from build123d import *

# Parameters (mm, degrees)
F_0_5IN_SOCKET_R    = 27.94
F_0_5IN_SOCKET_R_2  = 2.1
BOSS_EXTRUDE1_DEPTH = 6.35


with BuildPart() as part:
    # 0.5in Socket → Boss-Extrude1 (new body)
    with BuildSketch(Plane(origin=(0, 0, 0), x_dir=(1, 0, 0), z_dir=(0, 1, 0))):
        with Locations(Location((0, 0, 0), (0, 0, 270))):
            Circle(F_0_5IN_SOCKET_R)
        with Locations(Location((-14.997027722, -14.997027722, 0), (0, 0, 270))):
            Circle(F_0_5IN_SOCKET_R_2, mode=Mode.SUBTRACT)
        with Locations(Location((-14.997027722, 14.997027722, 0), (0, 0, 270))):
            Circle(F_0_5IN_SOCKET_R_2, mode=Mode.SUBTRACT)
        with Locations(Location((14.997027722, 14.997027722, 0), (0, 0, 270))):
            Circle(F_0_5IN_SOCKET_R_2, mode=Mode.SUBTRACT)
        with Locations(Location((14.997027722, -14.997027722, 0), (0, 0, 270))):
            Circle(F_0_5IN_SOCKET_R_2, mode=Mode.SUBTRACT)
        with BuildLine():
            ThreePointArc((2.530034488, -14.126221239), (0, -16.891), (-2.530034488, -14.126221239))
            ThreePointArc((-2.530034488, -14.126221239), (-14.351, 0), (-2.530034488, 14.126221239))
            ThreePointArc((-2.530034488, 14.126221239), (0, 16.891), (2.530034488, 14.126221239))
            ThreePointArc((2.530034488, 14.126221239), (14.351, 0), (2.530034488, -14.126221239))
        make_face(mode=Mode.SUBTRACT)
    extrude(amount=BOSS_EXTRUDE1_DEPTH)


solid = part.part
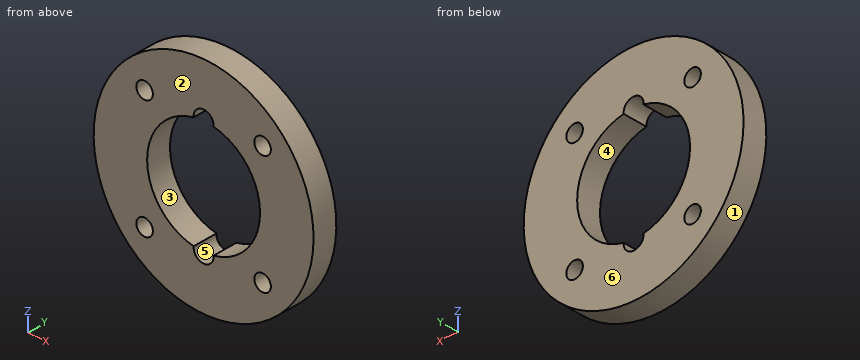
Read the model definition and answer for the solid it produces. Units are mm, in the model's axes. Face numbers are marked on the shaded views. A direction names the side the tool comes from. Round coordinates to 2 decimals unless told otherwise and drop trailing zeros. Order: outer loops, then holes, each group sorted by start corner. A loop starts at its lowest first (then second) coordinate and runs counter-clockwise, first axis right, second up. Notation, with made-up numbers: (-34, 64.5) - (-22, 64.5) arc R19 ccw to (-22, 92.5) - close; hole circle Ø2 at (-35.5, 66). An arc over 180 degrees is marked (long way). Use one line per item in the form item = value. Start each with the question number.
(1) The part is cut by section A-A (x = 0). Give the vertices of the cut face in (y, z).
(2) The part is cut by section D-D (x = 16). Give the vertices of the cut face in (y, z).
(3) The part is cut by section B-B (z = -10). Give the vertices of the cut face in (x, y).
(4) Flat-ended cylindrical pins translate along their axes: pin 1 Ø1.5 at (y, z) = (5.5, 7.5) entering from +X; pin 2 Ø1 at (x, y) = (-8, 4) entering from -Z; pin 3 Ø1.5 at (x, y) = (7.5, 2.5) entering from +Z; pin 4 Ø3 at (x, z) = (0, 14.351) entering from -Y. Find the tip coordinate at first contact, or state that the pin passes through.
(5) Determine the mould class of the marked faces 1, 2, 3 and 4 for opening direction Z: +Z half, -Z half, draft (parallel to the pull), parting line (faces both ways), or undercut.
(6) For the marked faces 5 and 6, determine the directions among +Z, -Z, +X, -X, +Y, -Y from which every point of the face is accessible in a straight line to the end or side of a thin tool.
(7) Find the intervals of material crossed by line 1 along X through (y, z) = (5.5, 0); line 2 along Z through (x, y) = (-15, 4.5); line 3 along X through (y, z) = (4.25, -3.5), in increasing order. Write a range as from..to.
(8) The part is cut by section C-C (y = 1.25). Give the vertices of the cut face in (x, z), then the cut area to 3 significant figures.
Checked values:
q1.outline = (0, -27.94) - (6.35, -27.94) - (6.35, -16.89) - (0, -16.89) - close; (0, 16.89) - (6.35, 16.89) - (6.35, 27.94) - (0, 27.94) - close
q2.outline = (0, -22.91) - (6.35, -22.91) - (6.35, -16.84) - (0, -16.84) - close; (0, -13.15) - (6.35, -13.15) - (6.35, 13.15) - (0, 13.15) - close; (0, 16.84) - (6.35, 16.84) - (6.35, 22.91) - (0, 22.91) - close
q3.outline = (-26.09, 0) - (-10.29, 0) - (-10.29, 6.35) - (-26.09, 6.35) - close; (10.29, 0) - (26.09, 0) - (26.09, 6.35) - (10.29, 6.35) - close
q4.pin_1 = 27.11
q4.pin_2 = -26.91
q4.pin_3 = 27.11
q4.pin_4 = through
q5.face_1 = parting line
q5.face_2 = draft
q5.face_3 = undercut
q5.face_4 = undercut
q6.face_5 = +Y, -Y
q6.face_6 = +Z, -Z, +X, -X, +Y
q7.line_1 = -27.94..-14.35, 14.35..27.94
q7.line_2 = -23.57..-17.1, -12.9..12.9, 17.1..23.57
q7.line_3 = -27.72..-13.92, 13.92..27.72
q8.outline = circle Ø55.88 at (0, 0); hole circle Ø4.2 at (-15, -15); hole circle Ø4.2 at (-15, 15); hole (-2.53, -14.13) arc R2.54 ccw (long way) to (2.53, -14.13) arc R14.35 ccw to (2.53, 14.13) arc R2.54 ccw (long way) to (-2.53, 14.13) arc R14.35 ccw to start; hole circle Ø4.2 at (15, -15); hole circle Ø4.2 at (15, 15)
q8.area = 1,730 mm^2
